Verification items for this drawing (mm, ordinates from the low corner). Coordinates: 2 decimals unless noted, no trailing zeros. Order: outer loops, then holes, each group sorted by start corner. A loop starts at its lowest first (then second) coordinate and runs counter-clockwise, first axis right, second up. Notation, with made-up numbers: M -29,18.25 L -13,18.25 A19 cw -13,34.25 Z; hole C 44,12 d10. An arc over 180 degrees is marked long. Write item = value, one per line.
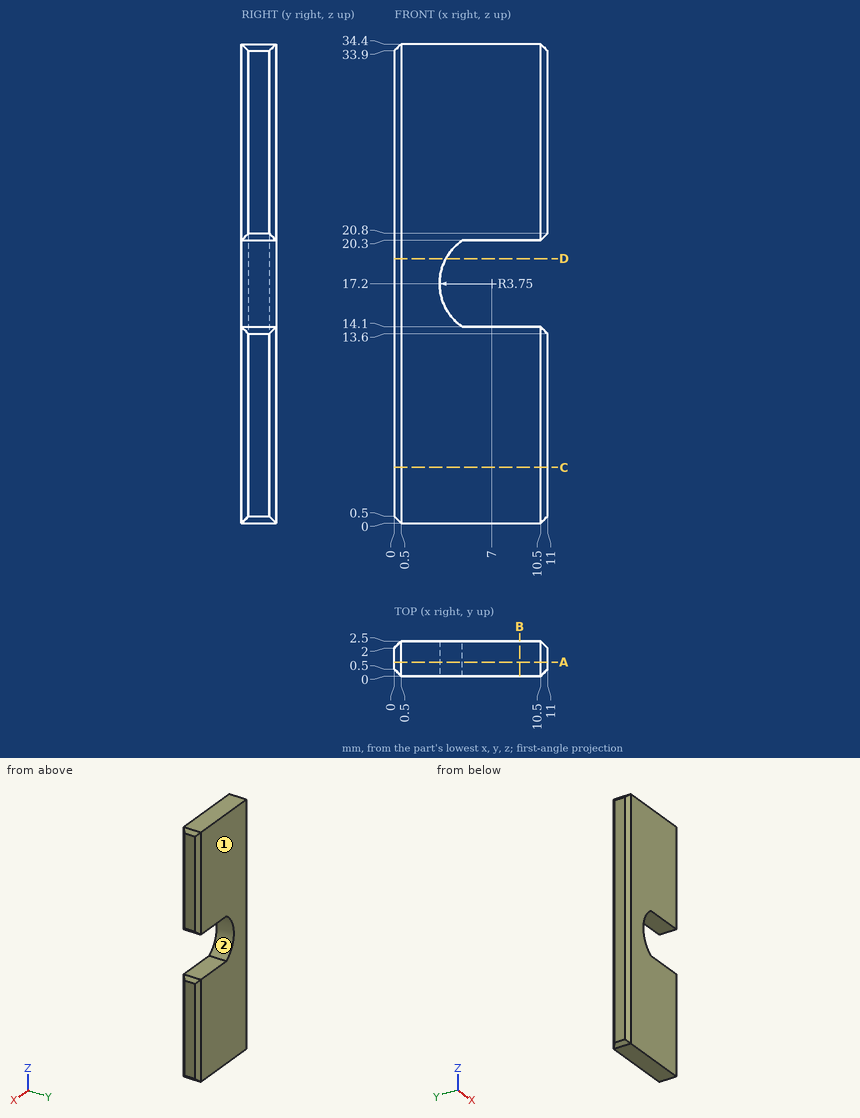
Item 1: Sectioned sample at C-C, the plane z = 4. Enter the section's corners in (x, y), then the cut area to 3 significant figures.
Report:
outline = M 0,0.5 L 0.5,0 L 10.5,0 L 11,0.5 L 11,2 L 10.5,2.5 L 0.5,2.5 L 0,2 Z
area = 27.0 mm^2
Item 2: Release check for a two-part mould opening along Z. For the marked faces 1 and 2 record: pulls with the +Z half, pulls with the -Z half, needs draft (parallel to the pull), parting line crosses it, or undercut.
Report:
face_1 = needs draft
face_2 = undercut
Item 3: Sectioned sample at B-B, the plane x = 9. Enter the section's corners in (y, z), then the cut area to 3 significant figures.
Report:
outline = M 0,0 L 2.5,0 L 2.5,14.1 L 0,14.1 Z; M 0,20.3 L 2.5,20.3 L 2.5,34.4 L 0,34.4 Z
area = 70.5 mm^2
Item 4: Sectioned sample at A-A, the plane y = 1. Enter the section's corners in (x, z).
Report:
outline = M 0,0.5 L 0.5,0 L 10.5,0 L 11,0.5 L 11,13.6 L 10.5,14.1 L 4.89,14.1 A3.75 cw 4.89,20.3 L 10.5,20.3 L 11,20.8 L 11,33.9 L 10.5,34.4 L 0.5,34.4 L 0,33.9 Z
Item 5: Sectioned sample at D-D, the plane z = 19. Enter the section's corners in (x, y), then the cut area to 3 significant figures.
Report:
outline = M 0,0.5 L 0.5,0 L 3.71,0 L 3.71,2.5 L 0.5,2.5 L 0,2 Z
area = 9.03 mm^2
Item 6: Scan lines: L1, parallel to Z at x = 8.25, y = 0.95; L2, parallel to Z at x = 4, y = 2.4; L3, parallel to X at y = 0.25, z = 12.5. Record each from-to range of solid material in increasing order. Write a range as from..to.
Report:
L1 = 0..14.1, 20.3..34.4
L2 = 0..14.95, 19.45..34.4
L3 = 0.25..10.75
